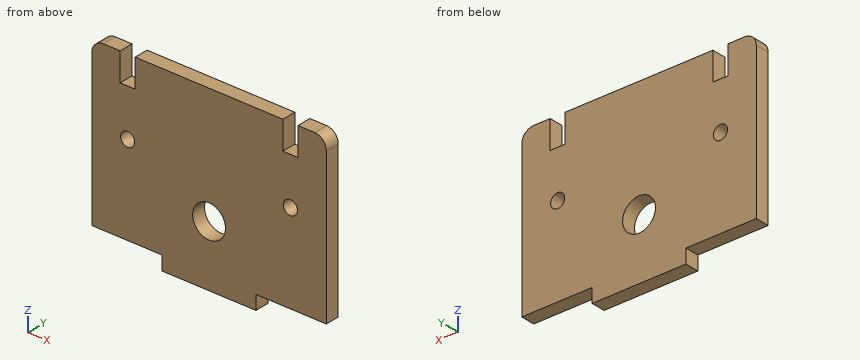
```python
from build123d import *

# Parameters (mm, degrees)
CROQUIS1_R              = 1.5
CROQUIS1_R_2            = 3.5
SALIENTE_EXTRUIR1_DEPTH = 3
CROQUIS4_W              = 20
CROQUIS4_H              = 3
SALIENTE_EXTRUIR2_DEPTH = 3


with BuildPart() as part:
    # Croquis1 → Saliente-Extruir1 (new body)
    with BuildSketch(Plane(origin=(0, 0, 0), x_dir=(1, 0, 0), z_dir=(0, 1, 0))):
        with BuildLine():
            Line((22.5, -17.5), (18.95, -17.5))
            Line((18.95, -17.5), (18.95, -11.5))
            Line((18.95, -11.5), (15.75, -11.5))
            Line((15.75, -11.5), (15.75, -17.5))
            Line((15.75, -17.5), (-15.75, -17.5))
            Line((-15.75, -17.5), (-15.75, -11.5))
            Line((-15.75, -11.5), (-18.95, -11.5))
            Line((-18.95, -11.5), (-18.95, -17.5))
            Line((-18.95, -17.5), (-22.5, -17.5))
            ThreePointArc((-22.5, -17.5), (-24.267766953, -16.767766953), (-25, -15))
            Line((-25, -15), (-25, 17.5))
            Line((-25, 17.5), (25, 17.5))
            Line((25, 17.5), (25, -15))
            ThreePointArc((25, -15), (24.267766953, -16.767766953), (22.5, -17.5))
        make_face()
        with Locations(Location((-17.35, -1.5, 0), (0, 0, 270))):
            Circle(CROQUIS1_R, mode=Mode.SUBTRACT)
        with Locations(Location((17.35, -1.5, 0), (0, 0, 90))):
            Circle(CROQUIS1_R, mode=Mode.SUBTRACT)
        with Locations(Location((0, 7.5, 0), (0, 0, 270))):
            Circle(CROQUIS1_R_2, mode=Mode.SUBTRACT)
    extrude(amount=SALIENTE_EXTRUIR1_DEPTH)

    # Croquis4 → Saliente-Extruir2 (add)
    with BuildSketch(Plane(origin=(0, 0, -17.5), x_dir=(-1, 0, 0), z_dir=(0, 0, -1))):
        with Locations((0, 1.5)):
            Rectangle(CROQUIS4_W, CROQUIS4_H)
    extrude(amount=SALIENTE_EXTRUIR2_DEPTH)


solid = part.part
```
Input: part model. Units: mm. Frame: model coordinates. Coordinates: 2 decimals unless noted, no trailing zeros. Loops run counter-clockwise (first coordinate to the right, second up) from the corner with the lowest first, then second, coordinate; pieces in that order, holes last.
Q1. Section D-D, the plane z = -7.5. Return the cut outline in (x, y), and give its area (3 significant figures).
Results are:
outline: (-25, 0) - (-3.5, 0) - (-3.5, 3) - (-25, 3) - close; (3.5, 0) - (25, 0) - (25, 3) - (3.5, 3) - close
area: 129 mm2
Q2. Section A-A, the plane x = 17.35. Return the cut outline in (y, z), and give its area (3 significant figures).
Results are:
outline: (0, -17.5) - (3, -17.5) - (3, 0) - (0, 0) - close; (0, 3) - (3, 3) - (3, 11.5) - (0, 11.5) - close
area: 78.0 mm2
Q3. Contact query for flat-ended pins moving along their axis: pin 1 (6.5 mm diameter, centred on x = 0, z = -7.5, fed in from -Y); pin 2 (0.9 mm diameter, centred on x = 17, y = 1.5, fed in from +Z); pin 3 (0.9 mm diameter, centred on x = -18.5, y = 1.5, fed in from -Z); pin 4 (1.5 mm diameter, centred on y = 1, z = -19, fed in from +X). Output: stop coordinate, or through.
Results are:
pin 1: passes through
pin 2: stops at z = 11.5
pin 3: stops at z = -17.5
pin 4: stops at x = 10
Q4. Line query: line 1 along X through (y, z) = (2.4, 13); line 2 along X through (y, z) = (2.35, 1.5); line 3 along X through (y, z) = (1, -7.5). Output: solid intervals per line, ascending.
Results are:
line 1: x = -25 to -18.95, -15.75 to 15.75, 18.95 to 25
line 2: x = -25 to -18.85, -15.85 to 15.85, 18.85 to 25
line 3: x = -25 to -3.5, 3.5 to 25
Q5. Section C-C, the plane y = 1.95. Return the cut outline in (x, z).
Results are:
outline: (-25, -17.5) - (-10, -17.5) - (-10, -20.5) - (10, -20.5) - (10, -17.5) - (25, -17.5) - (25, 15) arc R2.5 ccw to (22.5, 17.5) - (18.95, 17.5) - (18.95, 11.5) - (15.75, 11.5) - (15.75, 17.5) - (-15.75, 17.5) - (-15.75, 11.5) - (-18.95, 11.5) - (-18.95, 17.5) - (-22.5, 17.5) arc R2.5 ccw to (-25, 15) - close; hole circle Ø3 at (-17.35, 1.5); hole circle Ø7 at (0, -7.5); hole circle Ø3 at (17.35, 1.5)
Q6. Section B-B, the plane z = 1.5. Return the cut outline in (x, y), and give its area (3 significant figures).
Results are:
outline: (-25, 0) - (-18.85, 0) - (-18.85, 3) - (-25, 3) - close; (-15.85, 0) - (15.85, 0) - (15.85, 3) - (-15.85, 3) - close; (18.85, 0) - (25, 0) - (25, 3) - (18.85, 3) - close
area: 132 mm2
